from build123d import *

# Parameters (mm, degrees)
ESBO_O1_R                = 20
RESSALTO_EXTRUS_O1_DEPTH = 4.999999888


with BuildPart() as part:
    # Esboço1 → Ressalto-extrusão1 (new body)
    with BuildSketch(Plane(origin=(0, 0, 0), x_dir=(-1, 0, 0), z_dir=(0, 0, -1))):
        with Locations((48.763208571, 20.144551867)):
            Circle(ESBO_O1_R)
        with BuildLine():
            Line((47.645174582, 18.999999553), (49.881242559, 18.999999553))
            ThreePointArc((49.881242559, 18.999999553), (48.763208571, 21.744551867), (47.645174582, 18.999999553))
        make_face(mode=Mode.SUBTRACT)
        with BuildLine():
            Line((48.763208571, 24.144551867), (48.763208571, 35.144551867))
            ThreePointArc((48.763208571, 35.144551867), (38.156606853, 30.751153585), (33.763208571, 20.144551867))
            Line((33.763208571, 20.144551867), (44.763208571, 20.144551867))
            ThreePointArc((44.763208571, 20.144551867), (45.934781446, 22.972978992), (48.763208571, 24.144551867))
        make_face(mode=Mode.SUBTRACT)
        with BuildLine():
            Line((48.763208571, 5.144551867), (48.763208571, 16.144551867))
            ThreePointArc((48.763208571, 16.144551867), (51.591635695, 17.316124742), (52.763208571, 20.144551867))
            Line((52.763208571, 20.144551867), (63.763208571, 20.144551867))
            ThreePointArc((63.763208571, 20.144551867), (59.369810288, 9.537950149), (48.763208571, 5.144551867))
        make_face(mode=Mode.SUBTRACT)
    extrude(amount=-RESSALTO_EXTRUS_O1_DEPTH)


solid = part.part
Can you work these out from the model? Positions are in its coordinate system, mm. A direction names the side the tool comes from. Coordinates: 2 decimals unless noted, no trailing zeros. Loops run counter-clockwise (first coordinate to the right, second up) from the corner with the lowest first, then second, coordinate; pieces in that order, holes last. Notation, with made-up numbers: M -16.75,88.25 L 22.25,88.25 A29 ccw 22.25,114.25 Z; hole C 10,-9 d7. An arc over 180 degrees is marked long. Return JSON: item names as keys, results as strings. Group by question number.
Item 1: Imagine slicing it at B-B (y = 23.5). Please give me the cut outline in (x, z).
Item 2: Imagine slicing it at A-A (z = 2.8). Please give me the cut outline in (x, y), and give its area (3 significant figures).
Item 3: I'm going to push flat-ended pins straight in: pin 1 Ø1.5 at (x, z) = (-41.5, 2) entering from +Y; pin 2 Ø2.5 at (x, z) = (-59.5, 3.5) entering from -Y; pin 3 Ø0.7 at (x, z) = (-49, 3.5) entering from +Y. Where does each tip first touch, or does it pass through?
Item 4: Imagine slicing it at C-C (x = -59.5). Please give me the cut outline in (y, z).
Item 5: If I drill on L1, parallel to Y at x = -59.5, z = 3.15; L2, parallel to Y at x = -37.5, z = 2.4; L3, parallel to X at y = 15, z = 3.75, over which ranges is the centre line in solid material (lowest first)? Write a range as from..to.
Item 6: Imagine slicing it at D-D (x = -65.5). Please give me the cut outline in (y, z).
Item 7: On a 3-axis mill with a long thin cutter (end or side, diameter ignored), from which of +Z, -Z, +X, -X, +Y, -Y can I reach the whole of each face in a straight line? I mean faces 4 (the flat face through (-48, 16, 5)), 5 (the cylindrical face through (-59.49, 9.66, 2.46)). Say none if no direction works.
Item 8: Thinking about a two-plate mould opening in X: for faces 1 (the flat face through (-48, 16, 0)), 2 (the flat face through (-49, 19, 2)), 3 (the cylindrical face through (-28.783, 21.024, 2.465)), which applies, released by +X, released by -X, zero draft, split by the parting line, or undercut?
Verdict:
{
 "1": {"outline": "M -68.48,0 L -46.59,0 L -46.59,5 L -68.48,5 Z; M -34.14,0 L -29.05,0 L -29.05,5 L -34.14,5 Z"},
 "2": {"outline": "C -48.76,20.14 d40; hole M -63.76,20.14 A15 ccw -48.76,5.14 L -48.76,16.14 A4 cw -52.76,20.14 Z; hole M -49.88,19 L -47.65,19 A1.6 ccw long Z; hole M -48.76,24.14 A4 cw -44.76,20.14 L -33.76,20.14 A15 ccw -48.76,35.14 Z", "area": "921 mm^2"},
 "3": {"pin 1": "stops at y = 39.05", "pin 2": "stops at y = 2.54", "pin 3": "stops at y = 40.14"},
 "4": {"outline": "M 3.27,0 L 9.67,0 L 9.67,5 L 3.27,5 Z; M 20.14,0 L 37.02,0 L 37.02,5 L 20.14,5 Z"},
 "5": {"L1": "y = 3.27..9.67, 20.14..37.02", "L2": "y = 3.62..20.14, 30.05..36.67", "L3": "x = -68.09..-62.85, -48.76..-29.44"},
 "6": {"outline": "M 9.2,0 L 31.09,0 L 31.09,5 L 9.2,5 Z"},
 "7": {"face 4": "+Z, +X, -X, +Y, -Y", "face 5": "+Z, -Z"},
 "8": {"face 1": "zero draft", "face 2": "undercut", "face 3": "split by the parting line"}
}
